```python
from build123d import *

# Parameters (mm, degrees)
SKETCH1_W           = 1832
SKETCH1_H           = 100
BOSS_EXTRUDE1_DEPTH = 8
SKETCH2_W           = 8
SKETCH2_H           = 100
BOSS_EXTRUDE2_DEPTH = 88
BOSS_EXTRUDE3_DEPTH = 50
SKETCH4_W           = 620
SKETCH4_H           = 8
SKETCH4_W_2         = 310
BOSS_EXTRUDE4_DEPTH = 88


with BuildPart() as part:
    # Sketch1 → Boss-Extrude1 (new body)
    with BuildSketch(Plane.XY):
        Rectangle(SKETCH1_W, SKETCH1_H)
    extrude(amount=BOSS_EXTRUDE1_DEPTH)

    # Sketch2 → Boss-Extrude2 (add)
    with BuildSketch(Plane(origin=(0, 0, 0), x_dir=(-1, 0, 0), z_dir=(0, 0, -1))):
        with Locations((-912, 0)):
            Rectangle(SKETCH2_W, SKETCH2_H)
        with Locations((912, 0)):
            Rectangle(SKETCH2_W, SKETCH2_H)
        with Locations((824, 0)):
            Rectangle(SKETCH2_W, SKETCH2_H)
        with Locations((506, 0)):
            Rectangle(SKETCH2_W, SKETCH2_H)
        with Locations((314, 0)):
            Rectangle(SKETCH2_W, SKETCH2_H)
        with Locations((-4, 0)):
            Rectangle(SKETCH2_W, SKETCH2_H)
        with Locations((-196, 0)):
            Rectangle(SKETCH2_W, SKETCH2_H)
        with Locations((-824, 0)):
            Rectangle(SKETCH2_W, SKETCH2_H)
    extrude(amount=BOSS_EXTRUDE2_DEPTH)

    # Sketch3 → Boss-Extrude3 (add)
    with BuildSketch(Plane(origin=(0, 50, 0), x_dir=(1, 0, 0), z_dir=(0, 1, 0))):
        Polygon((-916, 88), (-916, -8), (-820, -8), (-820, 88), (-828, 88), (-828, 0), (-908, 0), (-908, 88), align=None)
        Polygon((-510, 88), (-510, -8), (-310, -8), (-310, 88), (-318, 88), (-318, 0), (-502, 0), (-502, 88), align=None)
        Polygon((0, 88), (0, -8), (200, -8), (200, 88), (192, 88), (192, 0), (8, 0), (8, 88), align=None)
        Polygon((820, 88), (820, -8), (916, -8), (916, 88), (908, 88), (908, 0), (828, 0), (828, 88), align=None)
    extrude(amount=BOSS_EXTRUDE3_DEPTH)

    # Sketch4 → Boss-Extrude4 (add)
    with BuildSketch(Plane(origin=(0, 0, 0), x_dir=(-1, 0, 0), z_dir=(0, 0, -1))):
        with Locations((-510, 46)):
            Rectangle(SKETCH4_W, SKETCH4_H)
        with Locations((155, 46)):
            Rectangle(SKETCH4_W_2, SKETCH4_H)
        with Locations((665, 46)):
            Rectangle(SKETCH4_W_2, SKETCH4_H)
    extrude(amount=BOSS_EXTRUDE4_DEPTH)


solid = part.part
```
Input: part model. Units: mm. Frame: model coordinates. A direction names the side the tool comes from. Round coordinates to 2 decimals unless told otherwise and drop trailing zeros. Loops run counter-clockwise (first coordinate to the right, second up) from the corner with the lowest first, then second, coordinate; pieces in that order, holes last. Notation, with made-up numbers: (89, 2) -> (114, 2) arc R18 cw to (114, 18) -> close; hole circle Ø10 at (14.25, -20.75). An arc over 180 degrees is marked (long way). Write each question's results on one line, items separated by ' | '.
1. First-contact query: P1, Ø8, axis at x = -517, y = 68.5, coming from the -Z side (3 decimals); P2, Ø1.5, axis at x = 215.5, z = -70.5, coming from the +Y side; P3, Ø3, axis at x = 248.5, z = -66.5, coming from the -Y side; P4, Ø5, axis at x = 355.5, y = -12, coming from the -Z side. Flat tips, straight axial feed; report the tip coordinate or a pass-through.
Geometry results:
P1: through | P2: y = 50 | P3: y = 42 | P4: z = 0
2. Section A-A (y = 74). State how many separate pieces and enclosed holes the cut face has, and give its area (3 significant figures).
Geometry results:
separate pieces: 4 | enclosed holes: 0 | area: 10,400 mm2
3. Ray query, line 1 (Z direction, x = 451.5, y = -30); line 2 (Y direction, x = 746.5, z = -82). Return the intervals inside material, ascending. Write a range as from..to.
Geometry results:
line 1: 0..8 | line 2: 42..50
4. Section B-B (x = -654.5). Return loops of the section in (y, z).
Geometry results:
outline: (-50, 0) -> (42, 0) -> (42, -88) -> (50, -88) -> (50, 8) -> (-50, 8) -> close
5. Section D-D (x = -393). Return loops of the section in (y, z).
Geometry results:
outline: (-50, 0) -> (100, 0) -> (100, 8) -> (-50, 8) -> close
6. Set-up query: faces 3 (the face through (-153, 42, -43)), 4 (the face through (-867, 24, 0)), 5 (the face through (-154, 48, -88)), 6 (the face through (-13, 7, 8)), 7 (the face through (-153, 50, -39)). Return all of +Z, -Z, +X, -X, +Y, -Y with unobstructed straight access to the full face (end or side cutting, diameter ignored); none if empty.
Geometry results:
face 3: -Z, -Y | face 4: -Z, +Y, -Y | face 5: -Z, +X, -X, +Y, -Y | face 6: +Z, +X, -X, +Y, -Y | face 7: +Z, -Z, +Y
7. Mould query, pull axis X, two halves, no side actions, for faces 1 (the face through (-663, 42, -43)), 2 (the face through (-868, 100, 2)). Classes: +X half, -X half, draft (parallel to the pull), parting line (faces both ways), or undercut.
Geometry results:
face 1: undercut | face 2: draft
